from build123d import *

# Parameters (mm, degrees)
BOSS_EXTRUDE1_DEPTH         = 1322.07
FILLET1_R                   = 1.27
BOSS_EXTRUDE2_DEPTH         = 2.54
F_1_4_0_25_DIAMETER_HOLE1_D = 6.35
F_1_4_CLEARANCE_HOLE1_D     = 6.7564


with BuildPart() as part:
    # Sketch1 → Boss-Extrude1 (new body)
    with BuildSketch(Plane(origin=(0, 0, 0), x_dir=(1, 0, 0), z_dir=(0, 1, 0))):
        Polygon((-9.225470009, 5.284705426), (-9.189424155, -5.347138677), (0.036045854, -10.631844103), (9.225470009, -5.284705426), (9.189424155, 5.347138677), (-0.036045854, 10.631844103), align=None)
        Polygon((-7.98301547, 4.502962617), (-7.891187754, -4.662012887), (0.091827716, -9.164975505), (7.98301547, -4.502962617), (7.891187754, 4.662012887), (-0.091827716, 9.164975505), align=None, mode=Mode.SUBTRACT)
    extrude(amount=BOSS_EXTRUDE1_DEPTH)

    # Fillet1
    fillet1_edges = [part.edges().sort_by_distance(p)[0] for p in [
        (-0.036045854, 661.035, -10.631844103),
        (9.189424155, 661.035, -5.347138677),
        (0.036045854, 661.035, 10.631844103),
        (-9.189424155, 661.035, 5.347138677),
        (-9.225470009, 661.035, -5.284705426),
        (7.98301547, 661.035, 4.502962617),
    ]]
    fillet(fillet1_edges, radius=FILLET1_R)

    # Sketch3 → Boss-Extrude2 (add)
    with BuildSketch(Plane.XZ):
        with BuildLine():
            Line((0.600193457, -10.26738166), (8.553184844, -5.71160112))
            ThreePointArc((8.553184844, -5.71160112), (9.019610446, -5.24832754), (9.191910076, -4.613908049))
            Line((9.191910076, -4.613908049), (9.225470009, 5.284705426))
            Line((9.225470009, 5.284705426), (0.669799244, 10.263075918))
            ThreePointArc((0.669799244, 10.263075918), (0.035379754, 10.435375548), (-0.600193457, 10.26738166))
            Line((-0.600193457, 10.26738166), (-8.553184844, 5.71160112))
            ThreePointArc((-8.553184844, 5.71160112), (-9.019610446, 5.24832754), (-9.191910076, 4.613908049))
            Line((-9.191910076, 4.613908049), (-9.222984088, -4.551474798))
            ThreePointArc((-9.222984088, -4.551474798), (-9.0549902, -5.187048009), (-8.591716619, -5.653473611))
            Line((-8.591716619, -5.653473611), (-0.669799244, -10.263075918))
            ThreePointArc((-0.669799244, -10.263075918), (-0.035379754, -10.435375548), (0.600193457, -10.26738166))
        make_face()
    extrude(amount=BOSS_EXTRUDE2_DEPTH)

    # 1/4 (0.25) Diameter Hole1 (through all)
    with Locations(Plane(origin=(0, -2.54, 0), x_dir=(-1, 0, 0), z_dir=(0, -1, 0))):
        with Locations((0, 0)):
            Hole(F_1_4_0_25_DIAMETER_HOLE1_D / 2)

    # 1/4 Clearance Hole1 (through all)
    with Locations(Plane(origin=(9.207563136, 0, 0.003013921), x_dir=(-0.003390348, 0, -0.999994253), z_dir=(0.999994253, 0, -0.003390348))):
        with Locations((0, 1309.37)):
            Hole(F_1_4_CLEARANCE_HOLE1_D / 2)


solid = part.part
Input: part model. Units: mm. Frame: model coordinates. Give positions to 0.01 mm unless a question says otherwise; leave off trailing zeros. Loops run counter-clockwise (first coordinate to the right, second up) from the corner with the lowest first, then second, coordinate; pieces in that order, holes last. Notation, with made-up numbers: M 62,26.5 L 111,26.5 A12 cw 111,47.5 Z; hole C 78.5,75 d6. An arc over 180 degrees is marked long. Use CSV: the item, a comma, the result in double quotes.
(1) Section A-A, the plane y = 325. Return loops of the section in (x, z), plus the area to 3 significant figures.
Outcome:
outline,"M -9.22,-4.55 A1.27 ccw -8.59,-5.65 L -0.67,-10.26 A1.27 ccw 0.6,-10.27 L 8.55,-5.71 A1.27 ccw 9.19,-4.61 L 9.23,5.28 L 0.67,10.26 A1.27 ccw -0.6,10.27 L -8.55,5.71 A1.27 ccw -9.19,4.61 Z; hole M -7.98,-4.5 L -0.09,-9.16 L 7.89,-4.66 L 7.98,3.77 A1.27 ccw 7.35,4.88 L 0.09,9.16 L -7.89,4.66 Z"
area,"75.1 mm²"
(2) Material intervals for L1, parallel to X at y = 1084, z = -4; L2, parallel to Z at x = 0, y = -1.55 (3 decimals); L3, parallel to Z at x = -0.25, y = 1037, sorted ascending. Write a range as [from, to].
Outcome:
L1,"x = [-9.22, -7.98], [7.9, 9.19]"
L2,"z = [-10.435, -3.175], [3.175, 10.435]"
L3,"z = [-10.42, -9.07], [8.97, 10.4]"
(3) Pin query (flat end, axial travel): P1, Ø1, axis at y = 292.5, z = -0.5, coming from the +X side; P2, Ø8, axis at y = 1039.5, z = 2.5, coming from the -X side; P3, Ø5, axis at x = 0, z = 0, coming from the -Y side; P4, Ø1, axis at x = 5.5, y = 636, coming from the +Z side. Return the tip coordinate at first contact, or that it passes through.
Outcome:
P1,"stops at x = 9.21"
P2,"stops at x = -9.21"
P3,"passes through"
P4,"stops at z = 7.74"
(4) Section B-B, the plane z = 0. Count the separate pieces of the cut face and the enclosed holes in it, plus the area to 3 significant figures.
Outcome:
separate pieces,"4"
enclosed holes,"0"
area,"3,370 mm²"
